Can you work these out from the model? Positions are in its coordinate system, mm. A direction names the side the tool comes from. Coordinates: 2 decimals unless noted, no trailing zeros. Order: outer loops, then holes, each group sorted by start corner. A loop starts at its lowest first (then second) coordinate and runs counter-clockwise, first axis right, second up. Notation, with made-up numbers: (52, -3) -> (92, -3) arc R13 cw to (92, 16) -> close; hole circle Ø10 at (-6, 54.5). An arc over 180 degrees is marked (long way). Write item = value, one per line.
```python
from build123d import *

# Parameters (mm, degrees)
BOSS_EXTRUDE1_DEPTH            = 15.875
CUT_EXTRUDE1_REACH             = 62.253
SKETCH2_W                      = 19.05
SKETCH2_H                      = 82
CUT_EXTRUDE2_REACH             = 101.98
SKETCH3_W                      = 8.128
SKETCH3_H                      = 53.92
CUT_EXTRUDE3_REACH             = 106.403
SKETCH4_W                      = 9.525
SKETCH4_H                      = 6.2
F_5_16_0_3125_DIAMETER_HOLE1_D = 7.9375
FILLET1_R                      = 3.175
FILLET2_R                      = 3.175


with BuildPart() as part:
    # Sketch1 → Boss-Extrude1 (new, symmetric)
    with BuildSketch(Plane.XY):
        Polygon((-6.2, 69.8), (-6.2, -6.2), (69.8, -6.2), (69.8, 0), (0, 69.8), align=None)
        Polygon((0, 60), (60, 0), (0, 0), align=None, mode=Mode.SUBTRACT)
    extrude(amount=BOSS_EXTRUDE1_DEPTH, both=True)

    # Sketch2 → Cut-Extrude1 (cut, up to next)
    with BuildSketch(Plane(origin=(34.9, 34.9, 0), x_dir=(0, 0, -1), z_dir=(0.7071067811865475, 0.7071067811865476, 0)), mode=Mode.PRIVATE) as cut_extrude1_sk1:
        Rectangle(SKETCH2_W, SKETCH2_H)
    cut_extrude1_tool1 = extrude(cut_extrude1_sk1.sketch, amount=-CUT_EXTRUDE1_REACH, mode=Mode.PRIVATE) & part.part
    add(cut_extrude1_tool1.solids().sort_by_distance((34.9, 34.9, 0))[0], mode=Mode.SUBTRACT)

    # Sketch3 → Cut-Extrude2 (cut, up to next)
    with BuildSketch(Plane(origin=(0, 0, 0), x_dir=(0, 0, -1), z_dir=(1, 0, 0)), mode=Mode.PRIVATE) as cut_extrude2_sk1:
        with Locations((0, 32.04)):
            Rectangle(SKETCH3_W, SKETCH3_H)
    cut_extrude2_tool1 = extrude(cut_extrude2_sk1.sketch, amount=-CUT_EXTRUDE2_REACH, mode=Mode.PRIVATE) & part.part
    add(cut_extrude2_tool1.solids().sort_by_distance((0, 32.04, 0))[0], mode=Mode.SUBTRACT)

    # Sketch4 → Cut-Extrude3 (cut, up to next)
    with BuildSketch(Plane(origin=(69.8, 0, 0), x_dir=(0, 0, -1), z_dir=(1, 0, 0)), mode=Mode.PRIVATE) as cut_extrude3_sk1:
        with Locations((-11.1125, -3.1)):
            Rectangle(SKETCH4_W, SKETCH4_H)
    cut_extrude3_tool1 = extrude(cut_extrude3_sk1.sketch, amount=-CUT_EXTRUDE3_REACH, mode=Mode.PRIVATE) & part.part
    # Sketch4 → Cut-Extrude3 (cut, up to next)
    with BuildSketch(Plane(origin=(69.8, 0, 0), x_dir=(0, 0, -1), z_dir=(1, 0, 0)), mode=Mode.PRIVATE) as cut_extrude3_sk2:
        with Locations((11.1125, -3.1)):
            Rectangle(SKETCH4_W, SKETCH4_H)
    cut_extrude3_tool2 = extrude(cut_extrude3_sk2.sketch, amount=-CUT_EXTRUDE3_REACH, mode=Mode.PRIVATE) & part.part
    add(cut_extrude3_tool1.solids().sort_by_distance((69.8, -3.1, 11.1125))[0], mode=Mode.SUBTRACT)
    add(cut_extrude3_tool2.solids().sort_by_distance((69.8, -3.1, -11.1125))[0], mode=Mode.SUBTRACT)

    # 5/16 (0.3125) Diameter Hole1 (through all)
    with Locations(Plane(origin=(0, -6.2, 0), x_dir=(-1, 0, 0), z_dir=(0, -1, 0))):
        with Locations((-31.8, 0)):
            Hole(F_5_16_0_3125_DIAMETER_HOLE1_D / 2)

    # Fillet1
    fillet1_edges = [part.edges().sort_by_distance(p)[0] for p in [
        (3.458621971, 61.441378029, 9.525),
        (61.441378029, 3.458621971, 9.525),
        (61.441378029, 3.458621971, -9.525),
        (3.458621971, 61.441378029, -9.525),
    ]]
    fillet(fillet1_edges, radius=FILLET1_R)

    # Fillet2
    fillet2_edges = [part.edges().sort_by_distance(p)[0] for p in [
        (-3.1, 59, -4.064),
        (-3.1, 5.08, -4.064),
        (-3.1, 5.08, 4.064),
        (-3.1, 59, 4.064),
    ]]
    fillet(fillet2_edges, radius=FILLET2_R)


solid = part.part
```
Item 1: I want a section at B-B, the plane y = 45. Please give me the cut outline in (x, z) (3 decimals), plus the area to 3 significant figures.
A:
outline = (-6.2, -15.875) -> (0, -15.875) -> (0, -4.064) -> (-6.2, -4.064) -> close; (-6.2, 4.064) -> (0, 4.064) -> (0, 15.875) -> (-6.2, 15.875) -> close; (15, -15.875) -> (24.8, -15.875) -> (24.8, -9.525) -> (15, -9.525) -> close; (15, 9.525) -> (24.8, 9.525) -> (24.8, 15.875) -> (15, 15.875) -> close
area = 271 mm2
Item 2: I want a section at A-A, the plane x = 31.8. Please give me the cut outline in (y, z) (3 decimals), plus the area to 3 significant figures.
A:
outline = (-6.2, -6.35) -> (0, -6.35) -> (0, -3.969) -> (-6.2, -3.969) -> close; (-6.2, 3.969) -> (0, 3.969) -> (0, 6.35) -> (-6.2, 6.35) -> close; (28.2, -15.875) -> (38, -15.875) -> (38, -9.525) -> (28.2, -9.525) -> close; (28.2, 9.525) -> (38, 9.525) -> (38, 15.875) -> (28.2, 15.875) -> close
area = 154 mm2
Item 3: I'm going to push flat-ended pins straight in: P1, Ø10.5, axis at x = 63.5, z = 13.5, coming from the -Y side; P2, Ø9.5, axis at y = 24.5, z = -4, coming from the +X side; P3, Ø7, axis at x = 34.5, y = -4.5, coming from the +Z side. Where does each tip first touch, or does it pass through?
A:
P1 = 0
P2 = 0
P3 = 6.35
Item 4: For faces 1 (the cylindrical face through (-3.143, 5.985, -3.109)), 2 (the flat face through (32, -3, 6.35)), 3 (the flat face through (-3, 59, 0)), which set-ups out of +Z, -Z, +X, -X, +Y, -Y let a thin tool reach every point of the face, with its end or its side?
A:
face_1 = -X
face_2 = +Z, +X, -X, -Y
face_3 = +X, -X
Item 5: I want a section at D-D, the plane z = 11. Please give me the cut outline in (x, y), plus the area to 3 significant figures.
A:
outline = (-6.2, 0) -> (0, 0) -> (0, 60) -> (60, 0) -> (69.8, 0) -> (0, 69.8) -> (-6.2, 69.8) -> close
area = 1,070 mm2
Item 6: If we mould it in two halves opening along Z, with no side actions, what happens to faces 4 (the cylindrical face through (60.767, 4.065, 8.57)), 5 (the flat face through (31.3, -6.2, -4.1)), 6 (the flat face through (32, -3, -6.35))? For each: pulls with the +Z half, pulls with the -Z half, needs draft (parallel to the pull), parting line crosses it, or undercut.
A:
face_4 = undercut
face_5 = needs draft
face_6 = pulls with the -Z half
Item 7: If I drill on probe 1 along Z at (x, y) = (31.8, -3.75); probe 2 along Z at (x, y) = (36, 25) (3 decimals); probe 3 along Y at (x, z) = (-2, 10), over which ranges is the centre line in solid material (lowest first)?
A:
probe_1 = -6.35 to -3.97, 3.97 to 6.35
probe_2 = -15.875 to -9.525, 9.525 to 15.875
probe_3 = 0 to 69.8
Item 8: I want a section at C-C, the plane x = 52. Please give me the cut outline in (y, z) (3 decimals).
A:
outline = (-6.2, -6.35) -> (0, -6.35) -> (0, 6.35) -> (-6.2, 6.35) -> close; (8, -15.875) -> (17.8, -15.875) -> (17.8, -9.525) -> (8, -9.525) -> close; (8, 9.525) -> (17.8, 9.525) -> (17.8, 15.875) -> (8, 15.875) -> close
